Autodesk Fusion 360 part; units mm, degrees
sketch "Sketch1" plane through (0, 0, 0) normal (0, 0, 1) x (1, 0, 0)
  line L0 (-27.3219, 46.2488) -> (22.1781, 46.2488)
  line L1 (28.1781, 40.2488) -> (28.1781, -47.2512)
  line L2 (22.1781, -53.2512) -> (-27.3219, -53.2512)
  line L3 (-33.3219, -47.2512) -> (-33.3219, 40.2488)
  arc A0 (28.1781, 40.2488) -> (22.1781, 46.2488) centre (22.1781, 40.2488) ccw
  arc A1 (-33.3219, -47.2512) -> (-27.3219, -53.2512) centre (-27.3219, -47.2512) ccw
  arc A2 (22.1781, -53.2512) -> (28.1781, -47.2512) centre (22.1781, -47.2512) ccw
  arc A3 (-27.3219, 46.2488) -> (-33.3219, 40.2488) centre (-27.3219, 40.2488) ccw
  arc A4 (22.1781, -55.2512) -> (30.1781, -47.2512) centre (22.1781, -47.2512) ccw
  line L4 (30.1781, 40.2488) -> (30.1781, -47.2512)
  arc A5 (30.1781, 40.2488) -> (22.1781, 48.2488) centre (22.1781, 40.2488) ccw
  line L5 (-27.3219, 48.2488) -> (22.1781, 48.2488)
  arc A6 (-27.3219, 48.2488) -> (-35.3219, 40.2488) centre (-27.3219, 40.2488) ccw
  line L6 (-35.3219, -47.2512) -> (-35.3219, 40.2488)
  arc A7 (-35.3219, -47.2512) -> (-27.3219, -55.2512) centre (-27.3219, -47.2512) ccw
  line L7 (22.1781, -55.2512) -> (-27.3219, -55.2512)
  line L8 (52.6781, 48.2488) -> (102.1781, 48.2488)
  line L9 (102.1781, -55.2512) -> (52.6781, -55.2512)
  line L10 (102.1781, -53.2512) -> (52.6781, -53.2512)
  arc A8 (102.1781, -53.2512) -> (108.1781, -47.2512) centre (102.1781, -47.2512) ccw
  line L11 (110.1781, 40.2488) -> (110.1781, -47.2512)
  arc A9 (46.6781, -47.2512) -> (52.6781, -53.2512) centre (52.6781, -47.2512) ccw
  line L12 (46.6781, -47.2512) -> (46.6781, 40.2488)
  line L13 (44.6781, -47.2512) -> (44.6781, 40.2488)
  arc A10 (108.1781, 40.2488) -> (102.1781, 46.2488) centre (102.1781, 40.2488) ccw
  arc A11 (52.6781, 46.2488) -> (46.6781, 40.2488) centre (52.6781, 40.2488) ccw
  arc A12 (52.6781, 48.2488) -> (44.6781, 40.2488) centre (52.6781, 40.2488) ccw
  arc A13 (44.6781, -47.2512) -> (52.6781, -55.2512) centre (52.6781, -47.2512) ccw
  arc A14 (102.1781, -55.2512) -> (110.1781, -47.2512) centre (102.1781, -47.2512) ccw
  arc A15 (110.1781, 40.2488) -> (102.1781, 48.2488) centre (102.1781, 40.2488) ccw
  line L14 (52.6781, 46.2488) -> (102.1781, 46.2488)
  line L15 (108.1781, 40.2488) -> (108.1781, -47.2512)
  line L16 (44.6781, 39.6601) -> (44.6781, -47.2512)
  line L17 (30.1781, -47.2512) -> (30.1781, 39.6601)
  line L18 (28.1781, 39.6696) -> (46.6781, 39.6696)
  line L19 (46.6781, 39.6696) -> (46.6781, -47.2512)
  line L20 (46.6781, -47.2512) -> (28.1781, -47.2512)
  line L21 (28.1781, -47.2512) -> (28.1781, 39.6696)
  line L22 (43.6781, -44.2512) -> (31.1781, -44.2512)
  line L23 (31.1781, -44.2512) -> (31.1781, 36.6696)
  line L24 (31.1781, 36.6696) -> (43.6781, 36.6696)
  line L25 (43.6781, 36.6696) -> (43.6781, -44.2512)
  point P0 (-33.3219, 46.2488)
  point P1 (28.1781, 46.2488)
  point P2 (-33.3219, -53.2512)
  point P3 (108.1781, 46.2488)
  point P4 (46.6781, -53.2512)
  point P5 (46.6781, 46.2488)
  point P6 (80, 0)
  dimension "d1" = 61.5
  dimension "d2" = 99.5
  dimension "d3" = 6
  dimension "d4" = 2
  dimension "d7" = 80
  dimension "d8" = 0
  dimension "d11" = 3
extrude "Extrude1" add sketch "Sketch1" along normal blind 3 contours L0 L1 L2 L3 A0 A1 A2 A3 A4 L4 A5 L5 A6 L6 A7 L7 L18 L20 | L1 L4 L17 L18 L20 L21 | L4 L13 L16 L17 L18 L20 | L12 L13 L16 L18 L19 L20 | L8 L9 L10 A8 L11 A9 L12 L13 A10 A11 A12 A13 A14 A15 L14 L15 L18 L20
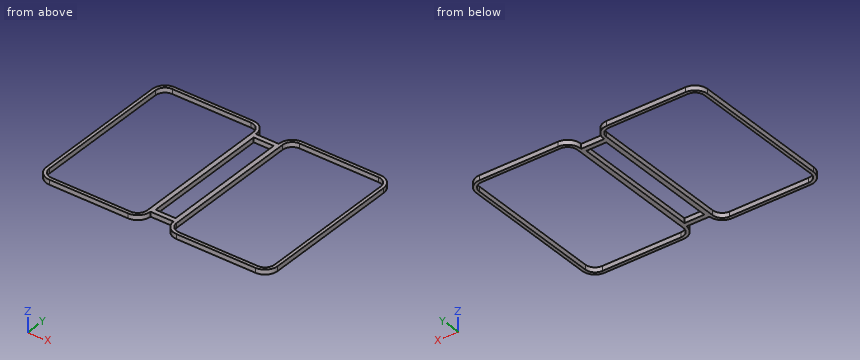
Work out the finished part from the listing and answer in its coordinate system (mm). Coordinates: 2 decimals unless noted, no trailing zeros. Order: outer loops, then holes, each group sorted by start corner. A loop starts at its lowest first (then second) coordinate and runs counter-clockwise, first axis right, second up. Notation, with made-up numbers: (44, -30) - (68, -30) arc R24 cw to (68, 4) - close; hole circle Ø7 at (-18.75, 22). An arc over 180 degrees is marked (long way). Put each result on its own line as item: value. Start each with the question number.
1) Find section D-D (x = 51). Give the vertices of the cut face in (y, z).
2) Find the intervals of material crossed by line 1 (X direction, y = 22, z = 1.1); line 2 (X direction, y = -46, z = 1.05); line 3 (Y direction, x = 40, z = 1.7), in increasing order. Write a range as from..to.
3) Find section B-B (y = -13). Give the vertices of the cut face in (x, z).
4) A flat-ended cylindrical pin translates along its axis: pin 1 (1.5 mm diameter, centred on x = 38, z = 1, fed in from -Y). Find the tip coordinate at first contact, or state that the pin passes through.
5) Find section C-C (z = 0.75). State how many separate pieces and enclosed holes the cut face has, plus the area to 3 significant figures.
6) Find section A-A (x = 14). Give the vertices of the cut face in (y, z), plus the area to 3 significant figures.
Results list:
1. outline: (-55.07, 0) - (-53.01, 0) - (-53.01, 3) - (-55.07, 3) - close; (46.01, 0) - (48.07, 0) - (48.07, 3) - (46.01, 3) - close
2. line 1: x = -35.32..-33.32, 28.18..31.18, 43.68..46.68, 108.18..110.18
2. line 2: x = -35.32..-33.32, 28.18..46.68, 108.18..110.18
2. line 3: y = -47.25..-44.25, 36.67..39.67
3. outline: (-35.32, 0) - (-33.32, 0) - (-33.32, 3) - (-35.32, 3) - close; (28.18, 0) - (31.18, 0) - (31.18, 3) - (28.18, 3) - close; (43.68, 0) - (46.68, 0) - (46.68, 3) - (43.68, 3) - close; (108.18, 0) - (110.18, 0) - (110.18, 3) - (108.18, 3) - close
4. pin 1: stops at y = -47.25
5. separate pieces: 1
5. enclosed holes: 3
5. area: 1,520 mm^2
6. outline: (-55.25, 0) - (-53.25, 0) - (-53.25, 3) - (-55.25, 3) - close; (46.25, 0) - (48.25, 0) - (48.25, 3) - (46.25, 3) - close
6. area: 12.0 mm^2
